Can you work these out from the drawing? Everything is in mm from the part's minimum corner. Give positions to 0.01 mm unless a question says otherwise; leave off trailing zeros. Write each loop counter-clockwise with the first axis right and the second up, starting at its lowest first coordinate (ties: lowest second). Pieces come first, ordered by that corner, then holes. Notation, with made-up numbers: (78.25, -19) - (116.25, -19) arc R12 ccw to (116.25, -6) - close; hole circle Ø11 at (52, -34). An arc over 180 degrees is marked (long way). Use a Markdown table: item, result. Add a question column.
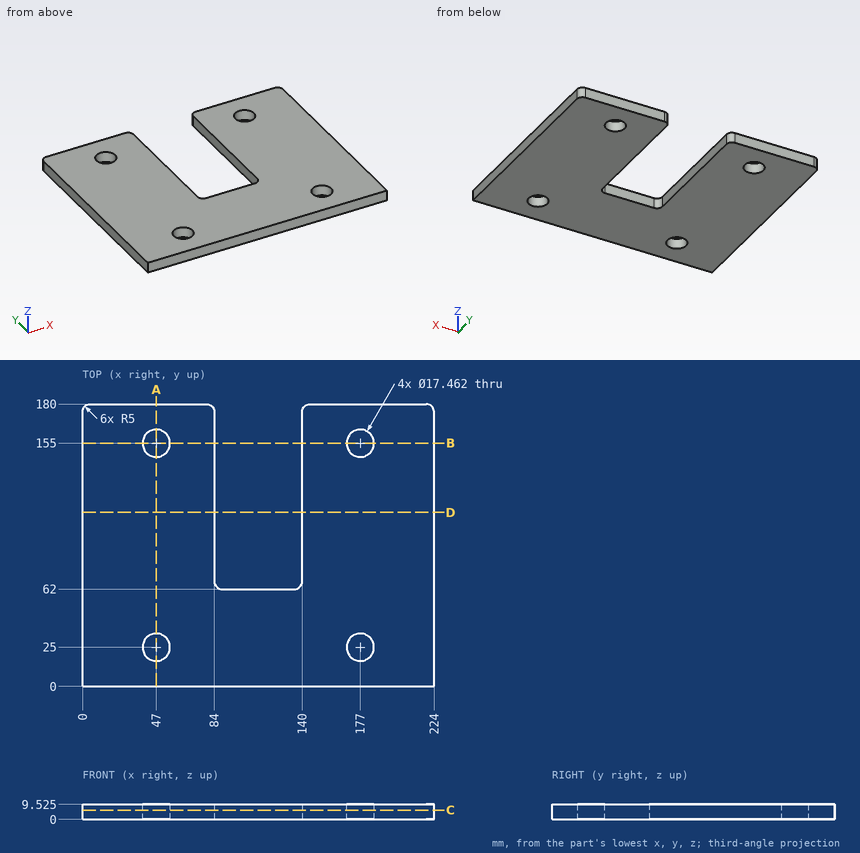
Q1. Suppose I cut it at D-D (y = 111). Please give me the cut outline in (x, z) (1 decimal).
Q2. Suppose I cut it at B-B (y = 155). Please give me the cut outline in (x, z) (1 decimal), and give its area (3 significant figures).
Q3. Suppose I cut it at A-A (x = 47). Please give me the cut outline in (y, z) (1 decimal), and give its area (3 significant figures).
Q4. Suppose I cut it at C-C (z = 6). Please give me the cut outline in (x, y), and give its area (3 significant figures).
Q5. If I drill on probe 1 along Y at (x, z) = (177, 3.5); probe 2 along X at (y, z) = (74, 0.5); probe 3 along Y at (x, z) = (173.5, 6), over which ranges is the centre line in solid material (lowest first)? Write a range as [from, to].
Q6. I'm going to push flat-ended pins straight in: P1, Ø3, axis at x = 132, z = 6.5, coming from the -Y side; P2, Ø10.5, axis at x = 47, y = 155, coming from the +Z side; P3, Ø3, axis at x = 140.5, z = 1, coming from the +Y side; P4, Ø3, axis at x = 111, z = 6.5, coming from the +Y side. Where does each tip first touch, or does it pass through?
Derived:
| question | item | result |
|---|---|---|
| 1 | outline | (0, 0) - (84, 0) - (84, 9.5) - (0, 9.5) - close; (140, 0) - (224, 0) - (224, 9.5) - (140, 9.5) - close |
| 2 | outline | (0, 0) - (38.3, 0) - (38.3, 9.5) - (0, 9.5) - close; (55.7, 0) - (84, 0) - (84, 9.5) - (55.7, 9.5) - close; (140, 0) - (168.3, 0) - (168.3, 9.5) - (140, 9.5) - close; (185.7, 0) - (224, 0) - (224, 9.5) - (185.7, 9.5) - close |
| 2 | area | 1,270 mm² |
| 3 | outline | (0, 0) - (16.3, 0) - (16.3, 9.5) - (0, 9.5) - close; (33.7, 0) - (146.3, 0) - (146.3, 9.5) - (33.7, 9.5) - close; (163.7, 0) - (180, 0) - (180, 9.5) - (163.7, 9.5) - close |
| 3 | area | 1,380 mm² |
| 4 | outline | (0, 0) - (224, 0) - (224, 175) arc R5 ccw to (219, 180) - (145, 180) arc R5 ccw to (140, 175) - (140, 67) arc R5 cw to (135, 62) - (89, 62) arc R5 cw to (84, 67) - (84, 175) arc R5 ccw to (79, 180) - (5, 180) arc R5 ccw to (0, 175) - close; hole circle Ø17.46 at (47, 25); hole circle Ø17.46 at (47, 155); hole circle Ø17.46 at (177, 25); hole circle Ø17.46 at (177, 155) |
| 4 | area | 32,700 mm² |
| 5 | probe 1 | [0, 16.27], [33.73, 146.27], [163.73, 180] |
| 5 | probe 2 | [0, 84], [140, 224] |
| 5 | probe 3 | [0, 17], [33, 147], [163, 180] |
| 6 | P1 | y = 0 |
| 6 | P2 | through |
| 6 | P3 | y = 179 |
| 6 | P4 | y = 62 |
